```python
from build123d import *

# Parameters (mm, degrees)
CROQUIS1_R              = 2.65
CROQUIS1_R_2            = 3.5
CROQUIS1_R_3            = 1.75
CROQUIS1_R_4            = 11.25
SALIENTE_EXTRUIR1_DEPTH = 6


with BuildPart() as part:
    # Croquis1 → Saliente-Extruir1 (new body)
    with BuildSketch(Plane.XY):
        Polygon((100, 100), (100, 0), (80, 0), (70, 10), (30, 10), (20, 0), (0, 0), (0, 100), (10, 110), (90, 110), align=None)
        with Locations((15, 70)):
            Circle(CROQUIS1_R, mode=Mode.SUBTRACT)
        with Locations((15, 10)):
            Circle(CROQUIS1_R_2, mode=Mode.SUBTRACT)
        with Locations((85, 10)):
            Circle(CROQUIS1_R_2, mode=Mode.SUBTRACT)
        with Locations((34.5, 100)):
            Circle(CROQUIS1_R_3, mode=Mode.SUBTRACT)
        with Locations((65.5, 100)):
            Circle(CROQUIS1_R_3, mode=Mode.SUBTRACT)
        with Locations((65.5, 69)):
            Circle(CROQUIS1_R_3, mode=Mode.SUBTRACT)
        with Locations((34.5, 69)):
            Circle(CROQUIS1_R_3, mode=Mode.SUBTRACT)
        with Locations((50, 84.5)):
            Circle(CROQUIS1_R_4, mode=Mode.SUBTRACT)
        with Locations((85, 70)):
            Circle(CROQUIS1_R, mode=Mode.SUBTRACT)
    extrude(amount=SALIENTE_EXTRUIR1_DEPTH)


solid = part.part
```
Work out the finished part from the listing and answer in its coordinate system (mm). A direction names the side the tool comes from. Coordinates: 2 decimals unless noted, no trailing zeros. Write each loop counter-clockwise with the first axis right and the second up, starting at its lowest first coordinate (ties: lowest second). Pieces come first, ordered by that corner, then holes.
Q1. A cutting plane is placed at A-A, the plane x = 15. Give the vertices of the cut face in (y, z).
Q2. Determine the mould class of faces 1 (the face through (75, 5, 3)), 2 (the face through (34.12, 67.29, 2.96)), 3 (the face through (95, 105, 3)), 4 (the face through (51, 56, 0)) for opening direction X: released by +X, released by -X, zero draft, split by the parting line, or undercut.
Q3. A cutting plane is placed at B-B, the plane x = 50. Give the vertices of the cut face in (y, z).
Q4. Which of the six approach directions +Z, -Z, +X, -X, +Y, -Y give full straight-line access (tool end or side, diameter ignored) to faces 5 (the face through (51, 56, 6)), 6 (the face through (50, 10, 3))?
Q5. A cutting plane is placed at D-D, the plane y = 89. Give the vertices of the cut face in (x, z), then the cut area to 3 significant figures.
Q6. A cutting plane is placed at C-C, the plane z = 2.1. State how many separate pieces and enclosed holes the cut face has, then the cut area to 3 significant figures.
Q7. Find the intervals of material crossed by line 1 (Y direction, x = 85, z = 3.95); line 2 (X direction, y = 100, z = 1.3); line 3 (X direction, y = 71, z = 1.4), in increasing order.
Q8. Each of these flat-tipped pins is pushed along its axis until it touches: pin 1 Ø4 at (x, y) = (15, 70) entering from -Z; pin 2 Ø3 at (x, z) = (40.5, 4) entering from -Y. Where does it stop, or does it pass through?
Findings below:
1. outline: (0, 0) - (6.5, 0) - (6.5, 6) - (0, 6) - close; (13.5, 0) - (67.35, 0) - (67.35, 6) - (13.5, 6) - close; (72.65, 0) - (110, 0) - (110, 6) - (72.65, 6) - close
2. face 1: undercut
2. face 2: undercut
2. face 3: released by +X
2. face 4: zero draft
3. outline: (10, 0) - (73.25, 0) - (73.25, 6) - (10, 6) - close; (95.75, 0) - (110, 0) - (110, 6) - (95.75, 6) - close
4. face 5: +Z, +X, -X, +Y, -Y
4. face 6: +Z, -Z, -Y
5. outline: (0, 0) - (39.69, 0) - (39.69, 6) - (0, 6) - close; (60.31, 0) - (100, 0) - (100, 6) - (60.31, 6) - close
5. area: 476 mm2
6. separate pieces: 1
6. enclosed holes: 9
6. area: 9,840 mm2
7. line 1: y = 0 to 6.5, 13.5 to 67.35, 72.65 to 110
7. line 2: x = 0 to 32.75, 36.25 to 63.75, 67.25 to 100
7. line 3: x = 0 to 12.55, 17.45 to 82.55, 87.45 to 100
8. pin 1: passes through
8. pin 2: stops at y = 10
